Verification items for the finished model (mm, model axes). A direction names the side the tool comes from. Give positions to 0.01 mm unless a question says otherwise; leave off trailing zeros. Order: outer loops, then holes, each group sorted by start corner. A loop starts at its lowest first (then second) coordinate and runs counter-clockwise, first axis right, second up.
Autodesk Inventor part; units mm, degrees
ref_plane "YZ Plane" through (0, 0, 0) normal (1, 0, 0) x (0, 1, 0)
ref_plane "XZ Plane" through (0, 0, 0) normal (0, 1, 0) x (-1, 0, 0)
ref_plane "XY Plane" through (0, 0, 0) normal (0, 0, 1) x (1, 0, 0)
sketch "Sketch1" plane through (0, 0, 0) normal (0, 0, 1) x (1, 0, 0)
  arc A0 (0, 5.15) -> (0, -5.15) centre (0, 0) ccw
  line L0 (0, 5.15) -> (0, 10)
  line L1 (0, -5.15) -> (0, -10)
  line L2 (0, 0) -> (-50, 0)
  line L3 (-50, 0) -> (-50, 25)
  line L4 (-50, 0) -> (-50, -25)
  line L5 (-50, -25) -> (0, -10)
  line L6 (-50, 25) -> (0, 10)
  line L7 (-50, 25) -> (-65, 25)
  line L8 (-65, 25) -> (-65, -25)
  line L9 (-65, -25) -> (-50, -25)
  line L10 (-50, 0) -> (-45, 0)
  line L11 (-45, 0) -> (-45, 23.5)
  line L12 (-45, 0) -> (-45, -23.5)
  line L13 (-5.15, 0) -> (-10.15, 0)
  line L14 (-10.15, 0) -> (-10.15, 13.045)
  line L15 (-10.15, 0) -> (-10.15, -13.045)
  line L16 (-45, -23.5) -> (-45, -18.5)
  line L17 (-45, -18.5) -> (-10.15, -8.045)
  line L18 (-45, 23.5) -> (-45, 18.5)
  line L19 (-45, 18.5) -> (-10.15, 8)
  line L20 (-57.5, 25) -> (-57.5, -25)
  line L21 (-65, 0) -> (-50, 0)
  line L22 (-65, 25) -> (-50, 10)
  line L23 (-65, 25) -> (-43.7868, 25) construction
  line L24 (-65, -25) -> (-50, -10)
  line L25 (-65, -25) -> (-43.7868, -25) construction
  circle A1 centre (-57.5, -17.5) radius 4.05
  circle A2 centre (-57.5, 17.5) radius 4.05
  dimension "d0" = 10.3
  dimension "d3" = 50
  dimension "d4" = 25
  dimension "d5" = 25
  dimension "d6" = 15
  dimension "d7" = 50
  dimension "d8" = 90
  dimension "d9" = 5
  dimension "d10" = 5
  dimension "d11" = 5
  dimension "d12" = 5
  dimension "d13" = 45
  dimension "d14" = 45
  dimension "d15" = 8.1
  dimension "d16" = 8.1
  dimension "d26" = 50
  dimension "d27" = 10
  dimension "d28" = 20
extrude "Extrusion1" add sketch "Sketch1" along normal blind 15 contours A0 L2 L14 L6 L0 | A0 L1 L5 L15 L2 | L14 L19 L11 L6 | L12 L5 L4 L2 | L2 L3 L6 L11 | L15 L5 L12 L17 | L21 L20 A2 L22 L3 | L4 L24 A1 L20 L21 | L3 L22 A2 L20 L7 | L4 L9 L20 A1 L24 | L21 L8 L22 A2 L20 | L20 A1 L24 L8 L21 | L20 A2 L22 L7 | L9 L24 A1 L20
sketch "Sketch2" plane through (-65, -25, 0) normal (-1, 0, 0) x (0, 0, 1)
  line L0 (0, 50) -> (0, 0)
  line L1 (0, 0) -> (15, 0)
  line L2 (15, 50) -> (15, 0)
  line L3 (0, 50) -> (15, 50)
  line L4 (0, 25) -> (15, 25)
  line L5 (7.5, 25) -> (7.5, 17.5)
  line L6 (7.5, 25) -> (7.5, 32.5)
  circle A0 centre (7.5, 32.5) radius 4.05
  circle A1 centre (7.5, 17.5) radius 4.05
  line L7 (7.5, 32.5) -> (11.55, 32.5)
  line L8 (11.55, 32.5) -> (11.55, 17.5)
  line L9 (7.5, 32.5) -> (3.45, 32.5)
  line L10 (3.45, 32.5) -> (3.45, 17.5)
  dimension "d19" = 7.5
  dimension "d20" = 7.5
  dimension "d21" = 8.1
  dimension "d22" = 8.1
extrude "Extrusion2" cut sketch "Sketch2" against normal up to surface (15 mm away) contours L10 A0 L6 L4 | L4 L5 A1 L10 | L6 A0 L8 L4 | L4 L8 A1 L5 | L9 L6 A0 | A0 L7 L9 | A1 | L6 L7 A0
fillet "Fillet1" radius 2 4 edges at (-45, -18.5, 7.5) (-10.15, -8.045, 7.5) (-45, 18.5, 7.5) (-10.15, 8, 7.5)
fillet "Fillet2" radius 2 2 edges at (-65, -25, 7.5) (-65, 25, 7.5)
properties part number "Rod_support_1"
(1) Section check D-D, the plane x = -19.5. Enter the section's corners in (y, z).
Solved:
outline: (-15.85, 0) - (-10.85, 0) - (-10.85, 15) - (-15.85, 15) - close; (10.82, 0) - (15.85, 0) - (15.85, 15) - (10.82, 15) - close
(2) Set-up check for faces 4 (the flat face through (-58, 0, 11.55)), 5 (the flat face through (-27.21, 13.14, 7.4)), 6 (the flat face through (-47, 0, 0)): record each of +Z, -Z, +X, -X, +Y, -Y from which the full face is reachable in a straight line by a thin tool's end or side.
Solved:
face 4: -X
face 5: +Z, -Z
face 6: -Z, +X, -X, +Y, -Y
(3) Section check C-C, the plane y = 0. Enter the section's corners in (x, z), then the cut area to 4 significant figures.
Solved:
outline: (-65, 0) - (-45, 0) - (-45, 15) - (-65, 15) - (-65, 11.55) - (-50, 11.55) - (-50, 3.45) - (-65, 3.45) - close; (-10.15, 0) - (-5.15, 0) - (-5.15, 15) - (-10.15, 15) - close
area: 253.5 mm2
(4) Release check for a two-part mould opening along X. For faces 1 (the cylindrical face through (-10.56, -7.77, 7.6)), 2 (the flat face through (0, 8, 7)), 3 (the flat face through (-57, -25, 7)) record: pulls with the +X half, pulls with the -X half, needs draft (parallel to the pull), parting line crosses it, or undercut.
Solved:
face 1: undercut
face 2: pulls with the +X half
face 3: needs draft
(5) Go/stop test with flat-tipped pins: pin 1 (6 mm diameter, centred on x = -7.5, z = 12.5, fed in from +Y); pin 2 (7.5 mm diameter, centred on x = -57.5, y = 17.5, fed in from +Z); pin 3 (5 mm diameter, centred on x = -23, z = 6, fed in from -Y); pin 4 (8 mm diameter, centred on x = -12, z = 3, fed in from +Y). Record where each tip stops, or that it passes through.
Solved:
pin 1: stops at y = 13.15
pin 2: passes through
pin 3: stops at y = -17.65
pin 4: stops at y = 14.8
(6) Section check A-A, the plane x = -57.5. Enter the section's corners in (y, z).
Solved:
outline: (-25, 0) - (-21.55, 0) - (-21.55, 15) - (-25, 15) - close; (-13.45, 0) - (13.45, 0) - (13.45, 15) - (-13.45, 15) - close; (21.55, 0) - (25, 0) - (25, 15) - (21.55, 15) - close; hole (-7.5, 3.45) - (7.5, 3.45) arc R4.05 ccw to (7.5, 11.55) - (-7.5, 11.55) arc R4.05 ccw to start
(7) Section check B-B, the plane z = 7.5. Enter the section's corners in (x, y).
Solved:
outline: (-65, -23) arc R2 ccw to (-63, -25) - (-50, -25) - (0, -10) - (0, -5.15) arc R5.15 cw to (0, 5.15) - (0, 10) - (-50, 25) - (-63, 25) arc R2 ccw to (-65, 23) - (-65, 11.55) - (-50, 11.55) - (-50, -11.55) - (-65, -11.55) - close; hole circle Ø8.1 at (-57.5, -17.5); hole circle Ø8.1 at (-57.5, 17.5); hole (-45, -15.81) arc R2 ccw to (-42.43, -17.73) - (-11.58, -8.47) arc R2 ccw to (-10.15, -6.56) - (-10.15, 6.51) arc R2 ccw to (-11.57, 8.43) - (-42.42, 17.72) arc R2 ccw to (-45, 15.81) - close
(8) Scan lines: line 1 (Y direction, x = -57.5, z = 5.5); line 2 (Y direction, x = -57.5, z = 4.75); line 3 (X direction, y = -6, z = 12). Record each from-to range of solid material in increasing order.
Solved:
line 1: y = -25 to -21.55, -13.45 to -11.02, 11.02 to 13.45, 21.55 to 25
line 2: y = -25 to -21.55, -13.45 to -10.47, 10.47 to 13.45, 21.55 to 25
line 3: x = -65 to -45, -10.15 to 0
